from build123d import *

# Parameters (mm, degrees)
F0_R            = 1.6
F0_W            = 20
F0_H            = 32.4
F1_DEPTH        = 3
F7_DEPTH        = 3
F9_DEPTH        = 3
F11_DEPTH       = 2.5
F12_D           = 3.5
F12_CSINK_D     = 5.5
F12_CSINK_ANGLE = 120
F14_W           = 24
F14_H           = 9.2
F15_DEPTH       = 15.5
F16_DEPTH       = 25


with BuildPart() as f1:
    # F0 (on Top) → F1 (new body)
    with BuildSketch(Plane.XY):
        with BuildLine():
            Line((-197.590603765, 7.6821263526), (-197.590603765, -13.9178736474))
            Line((-197.590603765, -13.9178736474), (-178.390603765, -13.9178736474))
            Line((-178.390603765, -13.9178736474), (-178.390603765, 8.7821263526))
            Line((-178.390603765, 8.7821263526), (-178.390603765, 17.3321263526))
            ThreePointArc((-178.390603765, 17.3321263526), (-179.740603765, 18.6821263526), (-178.390603765, 20.0321263526))
            Line((-178.390603765, 20.0321263526), (-178.390603765, 23.2821263526))
            ThreePointArc((-178.390603765, 23.2821263526), (-187.699120556, 19.8997481824), (-192.6648892104, 11.3306112011))
            ThreePointArc((-192.6648892104, 11.3306112011), (-193.3498228179, 10.1486612726), (-194.6337561684, 9.6821263526))
            Line((-194.6337561684, 9.6821263526), (-195.590603765, 9.6821263526))
            ThreePointArc((-195.590603765, 9.6821263526), (-197.0048173273, 9.096339915), (-197.590603765, 7.6821263526))
        make_face()
        with Locations((-183.390603765, 13.0821263526)):
            Circle(F0_R, mode=Mode.SUBTRACT)
        with BuildLine():
            Line((-178.390603765, -13.9178736474), (-197.590603765, -13.9178736474))
            Line((-197.590603765, -13.9178736474), (-197.590603765, -35.5178736474))
            ThreePointArc((-197.590603765, -35.5178736474), (-197.0048173273, -36.9320872098), (-195.590603765, -37.5178736474))
            Line((-195.590603765, -37.5178736474), (-194.6337561684, -37.5178736474))
            ThreePointArc((-194.6337561684, -37.5178736474), (-193.3498228179, -37.9844085674), (-192.6648892104, -39.1663584959))
            ThreePointArc((-192.6648892104, -39.1663584959), (-187.699120556, -47.7354954773), (-178.390603765, -51.1178736474))
            Line((-178.390603765, -51.1178736474), (-178.390603765, -47.8678736474))
            ThreePointArc((-178.390603765, -47.8678736474), (-179.740603765, -46.5178736474), (-178.390603765, -45.1678736474))
            Line((-178.390603765, -45.1678736474), (-178.390603765, -13.9178736474))
        make_face()
        with Locations((-183.390603765, -40.9178736474)):
            Circle(F0_R, mode=Mode.SUBTRACT)
        with BuildLine():
            Line((-178.390603765, 8.7821263526), (-178.390603765, -13.9178736474))
            Line((-178.390603765, -13.9178736474), (-161.890603765, -13.9178736474))
            Line((-161.890603765, -13.9178736474), (-161.890603765, 6.7821263526))
            ThreePointArc((-161.890603765, 6.7821263526), (-163.3048173273, 7.3679127902), (-163.890603765, 8.7821263526))
            Line((-163.890603765, 8.7821263526), (-178.390603765, 8.7821263526))
        make_face()
        with BuildLine():
            Line((-161.890603765, -13.9178736474), (-178.390603765, -13.9178736474))
            Line((-178.390603765, -13.9178736474), (-178.390603765, -45.1678736474))
            ThreePointArc((-178.390603765, -45.1678736474), (-177.4360096104, -45.5632794928), (-177.040603765, -46.5178736474))
            ThreePointArc((-177.040603765, -46.5178736474), (-177.4360096104, -47.472467802), (-178.390603765, -47.8678736474))
            Line((-178.390603765, -47.8678736474), (-178.390603765, -51.1178736474))
            ThreePointArc((-178.390603765, -51.1178736474), (-168.1375554378, -46.8709219746), (-163.890603765, -36.6178736474))
            ThreePointArc((-163.890603765, -36.6178736474), (-163.3048173273, -35.203660085), (-161.890603765, -34.6178736474))
            Line((-161.890603765, -34.6178736474), (-161.890603765, -13.9178736474))
        make_face()
        with Locations((-173.390603765, -40.9178736474)):
            Circle(F0_R, mode=Mode.SUBTRACT)
        Polygon((-161.890603765, 6.7821263526), (-161.890603765, -13.9178736474), (-121.890603765, -13.9178736474), (-121.890603765, 18.4821263526), align=None)
        Polygon((-121.890603765, -13.9178736474), (-161.890603765, -13.9178736474), (-161.890603765, -34.6178736474), (-121.890603765, -46.3178736474), align=None)
        with BuildLine():
            Line((-178.390603765, 17.3321263526), (-178.390603765, 8.7821263526))
            Line((-178.390603765, 8.7821263526), (-163.890603765, 8.7821263526))
            ThreePointArc((-163.890603765, 8.7821263526), (-168.1375554378, 19.0351746798), (-178.390603765, 23.2821263526))
            Line((-178.390603765, 23.2821263526), (-178.390603765, 20.0321263526))
            ThreePointArc((-178.390603765, 20.0321263526), (-177.4360096104, 19.6367205072), (-177.040603765, 18.6821263526))
            ThreePointArc((-177.040603765, 18.6821263526), (-177.4360096104, 17.727532198), (-178.390603765, 17.3321263526))
        make_face()
        with Locations((-173.390603765, 13.0821263526)):
            Circle(F0_R, mode=Mode.SUBTRACT)
        with Locations((-111.890603765, 2.2821263526)):
            Rectangle(F0_W, F0_H)
        with Locations((-111.890603765, -30.1178736474)):
            Rectangle(F0_W, F0_H)
        with BuildLine():
            Line((-101.890603765, 18.4821263526), (-101.890603765, -13.9178736474))
            Line((-101.890603765, -13.9178736474), (-81.890603765, -13.9178736474))
            Line((-81.890603765, -13.9178736474), (-81.890603765, -5.8178736474))
            Line((-81.890603765, -5.8178736474), (-81.890603765, 16.4821263526))
            ThreePointArc((-81.890603765, 16.4821263526), (-82.4763902026, 17.896339915), (-83.890603765, 18.4821263526))
            Line((-83.890603765, 18.4821263526), (-101.890603765, 18.4821263526))
        make_face()
        with BuildLine():
            Line((-81.890603765, -13.9178736474), (-101.890603765, -13.9178736474))
            Line((-101.890603765, -13.9178736474), (-101.890603765, -46.3178736474))
            Line((-101.890603765, -46.3178736474), (-83.890603765, -46.3178736474))
            ThreePointArc((-83.890603765, -46.3178736474), (-82.4763902026, -45.7320872098), (-81.890603765, -44.3178736474))
            Line((-81.890603765, -44.3178736474), (-81.890603765, -22.0178736474))
            Line((-81.890603765, -22.0178736474), (-81.890603765, -13.9178736474))
        make_face()
    extrude(amount=F1_DEPTH)

    # F6 (on plane+point) → F7 (join)
    with BuildSketch(Plane.XZ.offset(46.3178736474)):
        with BuildLine():
            Line((-98.890603765, 12.3), (-98.890603765, 0))
            Line((-98.890603765, 0), (-86.490603765, 0))
            Line((-86.490603765, 0), (-86.490603765, 12.3))
            Line((-86.490603765, 12.3), (-88.440603765, 12.3))
            ThreePointArc((-88.440603765, 12.3), (-92.690603765, 8.05), (-96.940603765, 12.3))
            Line((-96.940603765, 12.3), (-98.890603765, 12.3))
        make_face()
        with BuildLine():
            ThreePointArc((-86.490603765, 12.3), (-92.690603765, 18.5), (-98.890603765, 12.3))
            Line((-98.890603765, 12.3), (-96.940603765, 12.3))
            ThreePointArc((-96.940603765, 12.3), (-92.690603765, 16.55), (-88.440603765, 12.3))
            Line((-88.440603765, 12.3), (-86.490603765, 12.3))
        make_face()
    extrude(amount=-F7_DEPTH)

    # F8 (on plane+point) → F9 (join)
    with BuildSketch(Plane.XZ.offset(-18.4821263526)):
        with BuildLine():
            Line((-98.890603765, 12.3), (-98.890603765, 0))
            Line((-98.890603765, 0), (-86.490603765, 0))
            Line((-86.490603765, 0), (-86.490603765, 12.3))
            Line((-86.490603765, 12.3), (-88.440603765, 12.3))
            ThreePointArc((-88.440603765, 12.3), (-92.690603765, 8.05), (-96.940603765, 12.3))
            Line((-96.940603765, 12.3), (-98.890603765, 12.3))
        make_face()
        with BuildLine():
            ThreePointArc((-86.490603765, 12.3), (-92.690603765, 18.5), (-98.890603765, 12.3))
            Line((-98.890603765, 12.3), (-96.940603765, 12.3))
            ThreePointArc((-96.940603765, 12.3), (-92.690603765, 16.55), (-88.440603765, 12.3))
            Line((-88.440603765, 12.3), (-86.490603765, 12.3))
        make_face()
    extrude(amount=F9_DEPTH)

    # F10 (on plane+point) → F11 (join)
    with BuildSketch(Plane.XZ.offset(-8.4821263526)):
        with BuildLine():
            Line((-122.890603765, 22.3), (-122.890603765, 0))
            Line((-122.890603765, 0), (-101.490603765, 0))
            Line((-101.490603765, 0), (-101.490603765, 22.3))
            Line((-101.490603765, 22.3), (-107.8824719192, 22.3))
            ThreePointArc((-107.8824719192, 22.3), (-107.738829214, 21.6570413588), (-107.690603765, 21))
            ThreePointArc((-107.690603765, 21), (-109.0086232496, 17.8180194847), (-112.190603765, 16.5))
            ThreePointArc((-112.190603765, 16.5), (-115.3725842803, 17.8180194847), (-116.690603765, 21))
            ThreePointArc((-116.690603765, 21), (-116.6423783159, 21.6570413588), (-116.4987356107, 22.3))
            Line((-116.4987356107, 22.3), (-122.890603765, 22.3))
        make_face()
        with BuildLine():
            ThreePointArc((-112.190603765, 33), (-119.7566463237, 29.8660425587), (-122.890603765, 22.3))
            Line((-122.890603765, 22.3), (-116.4987356107, 22.3))
            ThreePointArc((-116.4987356107, 22.3), (-116.0520683136, 23.3106474287), (-115.3725842803, 24.1819805153))
            ThreePointArc((-115.3725842803, 24.1819805153), (-113.9126792106, 25.1574578963), (-112.190603765, 25.5))
            Line((-112.190603765, 25.5), (-112.190603765, 33))
        make_face()
        with BuildLine():
            Line((-107.8824719192, 22.3), (-101.490603765, 22.3))
            ThreePointArc((-101.490603765, 22.3), (-104.6245612063, 29.8660425587), (-112.190603765, 33))
            Line((-112.190603765, 33), (-112.190603765, 25.5))
            ThreePointArc((-112.190603765, 25.5), (-109.507322192, 24.6124783736), (-107.8824719192, 22.3))
        make_face()
    extrude(amount=F11_DEPTH)

    # F12 (through all)
    with Locations(Plane(origin=(0, 8.4821263526, 0), x_dir=(1, 0, 0), z_dir=(0, 1, 0))):
        with Locations((-106.1801961249, -27.0104076401), (-118.201011405, -14.9895923599)):
            CounterSinkHole(F12_D / 2, F12_CSINK_D / 2, counter_sink_angle=F12_CSINK_ANGLE)

    # F14 (on plane+point) → F15 (join)
    with BuildSketch(Plane.XZ.offset(7.3178736474)):
        with Locations((-110.890603765, 4.6)):
            Rectangle(F14_W, F14_H)
    extrude(amount=-F15_DEPTH)

    # F14 (on plane+point) → F16 (join)
    with BuildSketch(Plane.XZ.offset(7.3178736474)):
        with Locations((-110.890603765, 4.6)):
            Rectangle(F14_W, F14_H)
    extrude(amount=F16_DEPTH)


solid = f1.part
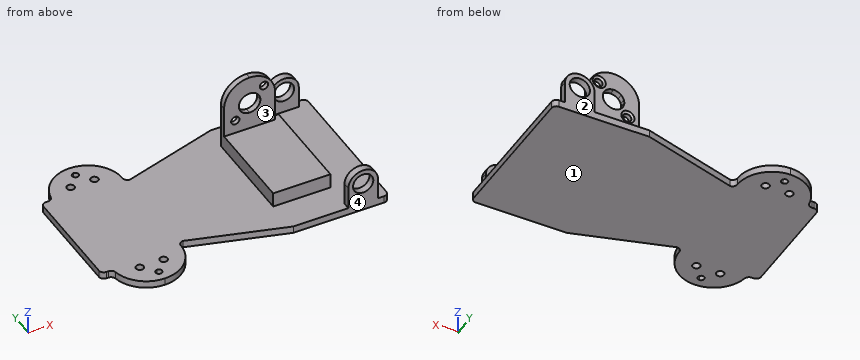
Model file for the job. Use its own axes, mm. Face numbers are marked on the shaded views. A direction names the side the tool comes from. Give positions to 0.01 mm unless a question says otherwise; leave off trailing zeros. Loops run counter-clockwise (first coordinate to the right, second up) from the corner with the lowest first, then second, coordinate; pieces in that order, holes last. Notation, with made-up numbers: (36, 87.5) - (77, 87.5) arc R21 ccw to (77, 121.5) - close; hole circle Ø2 at (-22, 12.5). An arc over 180 degrees is marked (long way). Use one line per item in the form item = value.
(1) Cut at A-A (y = -2). Give the cut face in (x, z), then the cut area to 3 significant figures.
Determined:
outline = (-197.59, 0) - (-81.89, 0) - (-81.89, 3) - (-98.89, 3) - (-98.89, 9.2) - (-122.89, 9.2) - (-122.89, 3) - (-197.59, 3) - close
area = 496 mm^2
(2) Cut at C-C (x = -170). Give the cut face in (y, z).
Determined:
outline = (-48.44, 0) - (20.61, 0) - (20.61, 3) - (-48.44, 3) - close
(3) 3-axis set-ups, long thin cutter, end or side, ignore diameter. For the marked faces 1, 2, 3 and 4: which of +Z, -Z, +X, -X, +Y, -Y reach the whole face in a straight line?
Determined:
face_1 = -Z, +X, -X, +Y, -Y
face_2 = +Z, -Z, +X, +Y
face_3 = +Z, +X, -X, -Y
face_4 = +Z, -Z, +X, -Y
(4) Drop flat-ended pins along their axis: P1, Ø3.5, axis at x = -183.39, y = -40.92, coming from the +Z side; P2, Ø3, axis at x = -111.5, z = 5.5, coming from the -Y side; P3, Ø10, axis at x = -170, z = 5, coming from the +Y side. Give the stop position or say it passes through.
Determined:
P1 = 3
P2 = -32.32
P3 = 22.77
(5) Cut at B-B (z = 11). Give the cut face in (x, y), then the cut area to 3 significant figures.
Determined:
outline = (-122.89, 5.98) - (-101.49, 5.98) - (-101.49, 8.48) - (-122.89, 8.48) - close; (-98.89, -46.32) - (-96.74, -46.32) - (-96.74, -43.32) - (-98.89, -43.32) - close; (-98.89, 15.48) - (-96.74, 15.48) - (-96.74, 18.48) - (-98.89, 18.48) - close; (-88.64, -46.32) - (-86.49, -46.32) - (-86.49, -43.32) - (-88.64, -43.32) - close; (-88.64, 15.48) - (-86.49, 15.48) - (-86.49, 18.48) - (-88.64, 18.48) - close
area = 79.3 mm^2
(6) Cut at D-D (x = -125). Give the cut face in (y, z), then the cut area to 3 significant figures.
Determined:
outline = (-45.41, 0) - (17.57, 0) - (17.57, 3) - (-45.41, 3) - close
area = 189 mm^2
(7) Drill centre lines: L1, parallel to Y at x = -97, z = 11; L2, parallel to Z at x = -137.5, y = -36.5; L3, parallel to Y at x = -107.5, z = 2.5. Where is each one in solid material? Low to high.
Determined:
L1 = -46.32 to -43.32, 15.48 to 18.48
L2 = 0 to 3
L3 = -46.32 to 18.48
